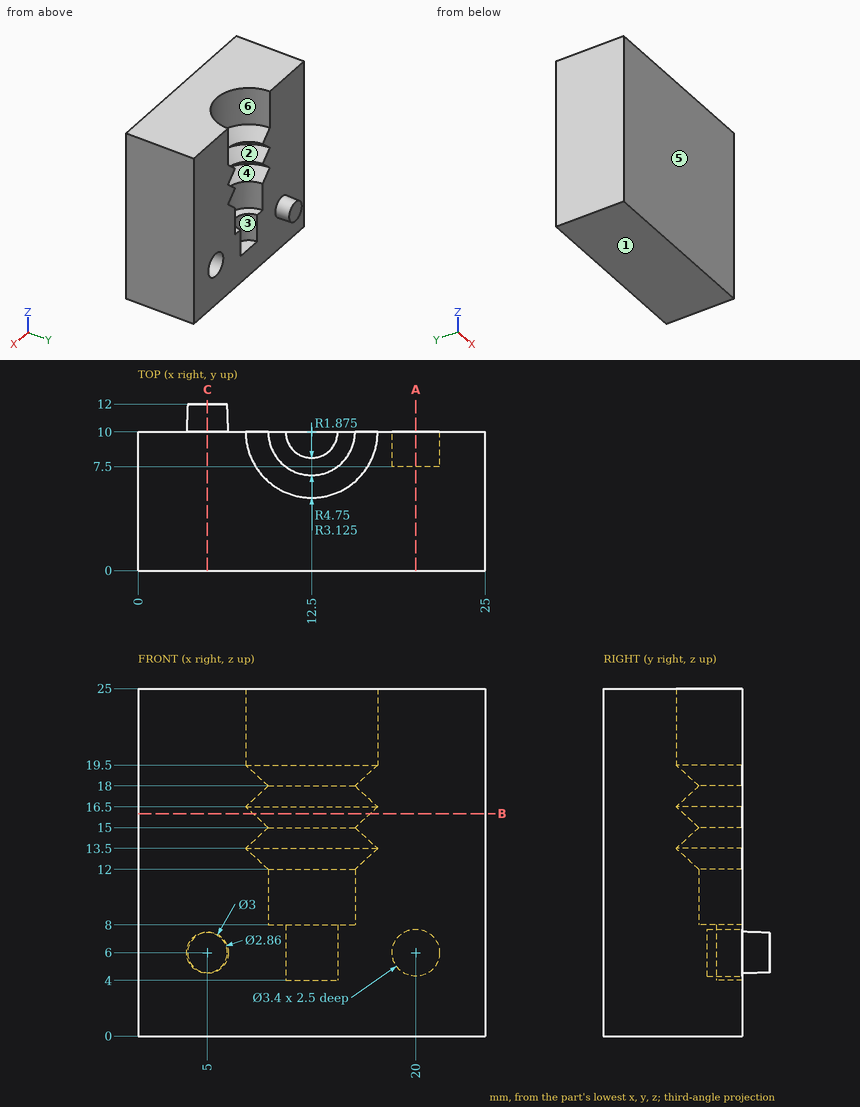
Geometry: see drawing. Coordinates: mm, zero at the bounding-box minimum. A direction names the side the tool comes from. Give positions to 0.01 mm unless a question says otherwise; leave off trailing zeros. Loops run counter-clockwise (first coordinate to the right, second up) from the corner with the lowest first, then second, coordinate; pieces in that order, holes last. Notation, with made-up numbers: (78, -10.5) - (85, -10.5) arc R25 ccw to (85, 27.5) - close; hole circle Ø5 at (5, -19.5). An arc over 180 degrees is marked (long way). Use CSV: the item, a comma, the result in double quotes. Start each with the question number.
1. Ray query, L1, parallel to Z at x = 20, y = 9.25; L2, parallel to X at y = 9.5, z = 7.5 (1 decimal); L3, parallel to X at y = 9.25, z = 7 (1 decimal). Return the intervals inside material, ascending.
2. Section B-B (z = 16). Output: boundary loops of the cut face in (x, y), then the cut area to 3 significant figures.
3. Section C-C (x = 5). Output: boundary loops of the cut face in (y, z), then the cut area to 3 significant figures.
4. Section A-A (x = 20). Output: boundary loops of the cut face in (y, z), then the cut area to 4 significant figures.
5. Pin query (flat end, axial travel): pin 1 (1 mm diameter, centred on x = 20, z = 5, fed in from +Y); pin 2 (1.6 mm diameter, centred on x = 12.5, y = 9, fed in from +Z); pin 3 (7.5 mm diameter, centred on x = 7.5, z = 17.5, fed in from +Y). Return the tip coordinate at first contact, or that it passes through.
6. Draft query along Z for the marked faces 1, 2, 3 and 4. Return one class per face: +Z half, -Z half, draft (parallel to the pull), parting line (faces both ways), or undercut.
7. Reachability of the marked faces 5 and 6 from +Z, -Z, +X, -X, +Y, -Y: full face, straight path, thin tool, end or side. Return the list, or none.
Response:
1,L1,"0 to 4.3, 7.7 to 25"
1,L2,"0 to 10.7, 14.3 to 19.2, 20.8 to 25"
1,L3,"0 to 10.8, 14.2 to 18.6, 21.4 to 25"
2,outline,"(0, 0) - (25, 0) - (25, 10) - (16.71, 10) arc R4.21 cw to (8.29, 10) - (0, 10) - close"
2,area,"222 mm²"
3,outline,"(0, 0) - (10, 0) - (10, 4.5) - (12, 4.57) - (12, 7.43) - (10, 7.5) - (10, 25) - (0, 25) - close"
3,area,"256 mm²"
4,outline,"(0, 0) - (10, 0) - (10, 4.3) - (7.5, 4.3) - (7.5, 7.7) - (10, 7.7) - (10, 25) - (0, 25) - close"
4,area,"241.5 mm²"
5,pin 1,"y = 7.5"
5,pin 2,"z = 4"
5,pin 3,"y = 10"
6,face 1,"-Z half"
6,face 2,"undercut"
6,face 3,"draft"
6,face 4,"undercut"
7,face 5,"+Z, -Z, +X, -X, -Y"
7,face 6,"+Z, +Y"
